```python
from build123d import *

# Parameters (mm, degrees)
SKETCH1_W           = 9
SKETCH1_H           = 5
BOSS_EXTRUDE1_DEPTH = 3
SKETCH2_RX          = 4.5
SKETCH2_RY          = 0.5727208
CUT_EXTRUDE1_DEPTH  = 10
FILLET1_START       = 30
FILLET1_DEPTH       = 7
CUT_EXTRUDE3_DEPTH  = 10
FILLET2_R           = 0.5
FILLET3_R           = 1


with BuildPart() as part:
    # Sketch1 → Boss-Extrude1 (new body)
    with BuildSketch(Plane(origin=(0, 0, 0), x_dir=(1, 0, 0), z_dir=(0, 1, 0))):
        with Locations((-89.22711343, -33.560593966)):
            Rectangle(SKETCH1_W, SKETCH1_H)
    extrude(amount=BOSS_EXTRUDE1_DEPTH)

    # Sketch2 → Cut-Extrude1 (cut)
    with BuildSketch(Plane.XY.offset(36.060593966)):
        with Locations((-89.22711343, 0)):
            Ellipse(SKETCH2_RX, SKETCH2_RY)
    extrude(amount=-CUT_EXTRUDE1_DEPTH, mode=Mode.SUBTRACT)

    # Fillet1: read off the stored shape, not the designer's step
    # Fillet1 outline → Fillet1 (cut)
    with BuildSketch(Plane.XY.offset(FILLET1_START)):
        with BuildLine():
            ThreePointArc((-84.72711343, 0.452186329), (-84.82937288, 0.250511517), (-85.052495268, 0.213821947))
            add(Edge.make_bspline(
                [(-84.72711343, 0), (-84.72711343, 0.110921166), (-85.052495268, 0.213821947)],
                knots=[0, 0, 0, 0.398284272, 0.398284272, 0.398284272], degree=2, weights=[1, 0.925735272, 0.889131025]))
            Line((-84.72711343, 0), (-84.72711343, 0.452186329))
        make_face()
        with BuildLine():
            ThreePointArc((-93.401731592, 0.213821947), (-93.62485398, 0.250511517), (-93.72711343, 0.452186329))
            Line((-93.72711343, 0.452186329), (-93.72711343, 0))
            add(Edge.make_bspline(
                [(-93.401731592, 0.213821947), (-93.72711343, 0.110921166), (-93.72711343, 0)],
                knots=[2.743308382, 2.743308382, 2.743308382, 3.141592654, 3.141592654, 3.141592654], degree=2, weights=[0.889131025, 0.925735272, 1]))
        make_face()
    extrude(amount=FILLET1_DEPTH, mode=Mode.SUBTRACT)

    # Sketch3 → Cut-Extrude3 (cut)
    with BuildSketch(Plane.XY.offset(36.060593966)):
        Polygon((-85.47711343, 2.0727208), (-85.47711343, 2.5727208), (-92.97711343, 2.5727208), (-92.97711343, 2.0727208), (-89.22711343, 2.0727208), align=None)
        Polygon((-88.82711343, 1.702215796), (-88.82711343, 1.102215796), (-89.62711343, 1.102215796), (-89.62711343, 1.702215796), (-89.22711343, 1.702215796), align=None)
    extrude(amount=-CUT_EXTRUDE3_DEPTH, mode=Mode.SUBTRACT)

    # Fillet2
    fillet2_edges = [part.edges().sort_by_distance(p)[0] for p in [
        (-84.72711343, 3, 33.560593966),
        (-93.72711343, 3, 33.560593966),
    ]]
    fillet(fillet2_edges, radius=FILLET2_R)

    # Fillet3
    # the kernel refuses this fillet: 1 mm, written as the material it takes off along each edge
    with BuildSketch(Plane(origin=(-85.47711343, 2.0727208, 31.060593966), x_dir=(0, -1, 0), z_dir=(-1, 0, 0)), Plane(origin=(-85.47711343, 2.0727208, 36.060593966), x_dir=(0, 0, -1), z_dir=(-1, 0, 0))) as fillet3_piece_1:
        with BuildLine():
            CenterArc((FILLET3_R, FILLET3_R), FILLET3_R, 180, 90)
            Line((0, FILLET3_R), (0, 0))
            Line((0, 0), (FILLET3_R, 0))
        make_face()
    extrude(amount=7.5, mode=Mode.SUBTRACT)


solid = part.part
```
Geometry check sheet. Reference: the model listing, model coordinates, mm. A direction names the side the tool comes from. Give positions to 0.01 mm unless a question says otherwise; leave off trailing zeros. Use a Markdown table: item, result.
Q1. Draft check along Y on faces 1 (the face through (-89, 3, 34)), 2 (the face through (-92.977, 2.3, 33.6)), 3 (the face through (-89.3, 2.8, 36.061)), 4 (the face through (-89, 2.573, 34)). Enter one of: pulls with the +Y half, pulls with the -Y half, needs draft (parallel to the pull), parting line crosses it, or undercut.
Computed:
| item | result |
|---|---|
| face 1 | pulls with the +Y half |
| face 2 | undercut |
| face 3 | needs draft |
| face 4 | undercut |
Q2. Section check B-B, the plane z = 33.6. Give the number of separate pieces and of enclosed holes in the cut face, then the cut area to 3 significant figures.
Computed:
| item | result |
|---|---|
| separate pieces | 1 |
| enclosed holes | 2 |
| area | 18.5 mm² |
Q3. Thickness scan on L1, parallel to X at y = 2.3, z = 35.55; L2, parallel to Y at x = -92, z = 32.05; L3, parallel to X at y = 1.5, z = 34.2. Record the ranges inside material, lowest first. Write a range as [from, to].
Computed:
| item | result |
|---|---|
| L1 | x = [-93.73, -92.98], [-85.48, -84.73] |
| L2 | y = [0.45, 2.07], [2.57, 3] |
| L3 | x = [-93.73, -89.63], [-88.83, -84.73] |
Q4. Set-up check for faces 5 (the face through (-93.727, 1, 34)), 6 (the face through (-89.17, 1.89, 35.64)), 7 (the face through (-89, 2.073, 34)), 8 (the face through (-89.2, 1.9, 31.5)): record each of +Z, -Z, +X, -X, +Y, -Y from which the full face is reachable in a straight line by a thin tool's end or side.
Computed:
| item | result |
|---|---|
| face 5 | +Z, -Z, -X, +Y, -Y |
| face 6 | +Z |
| face 7 | +Z, -Z |
| face 8 | -Z |
